```python
from build123d import *

# Parameters (mm, degrees)
F1_DEPTH    = 0.8
F2_DEPTH    = 1
F3_T4_ANGLE = 24.0749520294
F4_R        = 0.2
F5_T1_DEPTH = 10.790585283


# Not quite as in the source:
# - a fillet or chamfer that OpenCascade refuses, or shapes differently, is made with other operations: its cross-section is extruded or revolved along the edge and cut away or added


with BuildPart() as f1:
    # F0 (on Top) → F1 (new body)
    with BuildSketch(Plane.XY):
        with BuildLine():
            Line((-10.2, 0), (-0.8, 0))
            ThreePointArc((-0.8, 0), (-0.2343145751, 0.2343145751), (0, 0.8))
            Line((0, 0.8), (0, 0.9915242061))
            ThreePointArc((0, 0.9915242061), (-5.5, 1.5), (-11, 0.9915242061))
            Line((-11, 0.9915242061), (-11, 0.8))
            ThreePointArc((-11, 0.8), (-10.7656854249, 0.2343145751), (-10.2, 0))
        make_face()
        with BuildLine():
            ThreePointArc((-11, 0.9915242061), (-5.5, 1.5), (0, 0.9915242061))
            Line((0, 0.9915242061), (0, 1.3315242061))
            ThreePointArc((0, 1.3315242061), (-5.5, 1.84), (-11, 1.3315242061))
            Line((-11, 1.3315242061), (-11, 0.9915242061))
        make_face()
        with BuildLine():
            ThreePointArc((-11, 1.3315242061), (-5.5, 1.84), (0, 1.3315242061))
            Line((0, 1.3315242061), (0, 5.55))
            Line((0, 5.55), (-0.2328427125, 5.7828427125))
            ThreePointArc((-0.2328427125, 5.7828427125), (-0.319551813, 5.912612052), (-0.35, 6.0656854249))
            Line((-0.35, 6.0656854249), (-0.35, 6.9))
            ThreePointArc((-0.35, 6.9), (-0.2914213562, 7.0414213562), (-0.15, 7.1))
            Line((-0.15, 7.1), (-0.1, 7.1))
            ThreePointArc((-0.1, 7.1), (-0.0292893219, 7.1292893219), (0, 7.2))
            Line((0, 7.2), (0, 8.4343145751))
            ThreePointArc((0, 8.4343145751), (-0.030448187, 8.587387948), (-0.1171572875, 8.7171572875))
            Line((-0.1171572875, 8.7171572875), (-1.1828427125, 9.7828427125))
            ThreePointArc((-1.1828427125, 9.7828427125), (-1.269551813, 9.912612052), (-1.3, 10.0656854249))
            Line((-1.3, 10.0656854249), (-1.3, 14.2))
            ThreePointArc((-1.3, 14.2), (-1.5343145751, 14.7656854249), (-2.1, 15))
            Line((-2.1, 15), (-10.2, 15))
            ThreePointArc((-10.2, 15), (-10.7656854249, 14.7656854249), (-11, 14.2))
            Line((-11, 14.2), (-11, 1.3315242061))
        make_face()
    extrude(amount=F1_DEPTH)

    # F0 (on Top) → F2 (join)
    with BuildSketch(Plane.XY):
        with BuildLine():
            Line((-10.2, 0), (-0.8, 0))
            ThreePointArc((-0.8, 0), (-0.2343145751, 0.2343145751), (0, 0.8))
            Line((0, 0.8), (0, 0.9915242061))
            ThreePointArc((0, 0.9915242061), (-5.5, 1.5), (-11, 0.9915242061))
            Line((-11, 0.9915242061), (-11, 0.8))
            ThreePointArc((-11, 0.8), (-10.7656854249, 0.2343145751), (-10.2, 0))
        make_face()
    extrude(amount=F2_DEPTH)

    # F3: chamfer of 0.3 on 1 edges, made by hand


with BuildPart() as f3_tool2:
    # F3_s3 → F3_t4 (revolve)
    with BuildSketch(Plane(origin=(-11.0738065014, -2.3613816897, 0), x_dir=(0, 0, 1), z_dir=(-0.9780114007, -0.2085514329, 0))):
        Polygon((0.8, 3.5737079623), (1.1, 3.2737079623), (0.8, 3.2737079623), align=None)
    revolve(axis=Axis((-5.5, -28.5, 0.8), (0, 0, -1)), revolution_arc=F3_T4_ANGLE)

    split(bisect_by=Plane.YZ.offset(-11), keep=Keep.TOP)

    split(bisect_by=Plane.YZ, keep=Keep.BOTTOM)

    split(bisect_by=Plane.XY.offset(1), keep=Keep.BOTTOM)


with BuildPart() as f1_1:
    add(f1.part)

    # F3_t1: union F3_tool2
    add(f3_tool2.part)

    # F4
    f4_edges = [f1_1.edges().sort_by_distance(p)[0] for p in [
        (-5.5, 1.8, 0.8),
        (-5.5, 1.6, 1),
    ]]
    fillet(f4_edges, radius=F4_R)

    # F5: chamfer of 0.52 x 0.3 on 1 edges, made by hand

    # F5_s2 → F5_t1 (cut)
    with BuildSketch(Plane.YZ.offset(-11.5452926415)):
        Polygon((15, 0.3), (14.48, 0), (15, 0), align=None)
    extrude(amount=F5_T1_DEPTH, mode=Mode.SUBTRACT)


solid = f1_1.part
```
Here's how the part is built. I have some questions about the finished solid (model axes, mm). Round coordinates to 2 decimals unless told otherwise and drop trailing zeros. Write each loop counter-clockwise with the first axis right and the second up, starting at its lowest first coordinate (ties: lowest second). Pieces come first, ordered by that corner, then holes.
Q1. Please list where these lines run through material, in increasing order: probe 1 along Z at (x, y) = (-9.5, 7.5); probe 2 along X at (y, z) = (6.25, 0.1); probe 3 along X at (y, z) = (11.5, 0.65).
Q2. If we section it at A-A on z = 0.55: Write out the boundary of the cut face in (x, y).
Q3. If we section it at B-B on x = -5.5: Write out the boundary of the cut face in (y, z), plus the area to 3 significant figures.
Q4. If we section it at D-D on y = 6.5: Write out the boundary of the cut face in (x, z).
Q5. Will this pin go through, and if not, where does the flat tip stop? P1, Ø0.6, axis at y = 12.5, z = 0.5, coming from the +X side.
Q6. If we section it at C-C on y = 4.75: Write out the boundary of the cut face in (x, z).
Answer below:
1. probe 1: z = 0 to 0.8
1. probe 2: x = -11 to -0.35
1. probe 3: x = -11 to -1.3
2. outline: (-11, 0.8) arc R0.8 ccw to (-10.2, 0) - (-0.8, 0) arc R0.8 ccw to (0, 0.8) - (0, 5.55) - (-0.23, 5.78) arc R0.4 cw to (-0.35, 6.07) - (-0.35, 6.9) arc R0.2 cw to (-0.15, 7.1) - (-0.1, 7.1) arc R0.1 ccw to (0, 7.2) - (0, 8.43) arc R0.4 ccw to (-0.12, 8.72) - (-1.18, 9.78) arc R0.4 cw to (-1.3, 10.07) - (-1.3, 14.2) arc R0.8 ccw to (-2.1, 15) - (-10.2, 15) arc R0.8 ccw to (-11, 14.2) - close
3. outline: (0, 0) - (14.48, 0) - (15, 0.3) - (15, 0.8) - (1.88, 0.8) arc R0.2 cw to (1.74, 0.86) - (1.66, 0.94) arc R0.2 ccw to (1.52, 1) - (0, 1) - close
3. area: 12.3 mm2
4. outline: (-11, 0) - (-0.35, 0) - (-0.35, 0.8) - (-11, 0.8) - close
5. P1: stops at x = -1.3
6. outline: (-11, 0) - (0, 0) - (0, 0.8) - (-11, 0.8) - close
